Geometry: final body of the model. Coordinates: model frame, mm. Give positions to 0.01 mm unless a question says otherwise; leave off trailing zeros. Write each loop counter-clockwise with the first axis right and the second up, starting at its lowest first coordinate (ties: lowest second). Pieces come first, ordered by that corner, then holes. Notation, with made-up numbers: (-39.5, 20) -> (19.5, 20) arc R28 cw to (19.5, 54) -> close; hole circle Ø4 at (16, 24). An arc over 180 degrees is marked (long way). Answer as a JSON object with one key per item and string values.
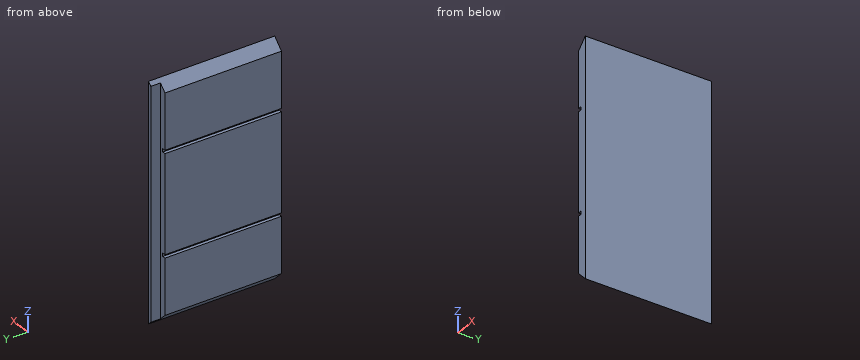
from build123d import *

# Parameters (mm, degrees)
F0_W     = 247.65
F0_H     = 457.2
F1_DEPTH = 19.05
F2_W     = 12.7
F2_H     = 19.05
F3_DEPTH = 457.201
F4_SIZE  = 19.04999
F5_SIZE  = 19.04999
F6_W     = 228.6
F6_H     = 6.35
F7_DEPTH = 6.35


# Not quite as in the source:
# - a fillet or chamfer is up to 0.001 mm smaller than in the source, because OpenCascade refuses the exact size


with BuildPart() as f1:
    # F0 (on Right) → F1 (new body)
    with BuildSketch(Plane.YZ):
        Rectangle(F0_W, F0_H)
    extrude(amount=F1_DEPTH)

    # F2 (on face) → F3 (cut, through all)
    with BuildSketch(Plane(origin=(0, 0, -228.6), x_dir=(1, 0, 0), z_dir=(0, 0, -1))):
        with Locations((6.35, -114.3)):
            Rectangle(F2_W, F2_H)
    extrude(amount=-F3_DEPTH, mode=Mode.SUBTRACT)

    # F4 (size 19.05 in the source; OpenCascade refuses exactly that, so slightly less here)
    f4_edges = [f1.edges().sort_by_distance(p)[0] for p in [
        (0, -9.525, 228.6),
    ]]
    chamfer(f4_edges, length=F4_SIZE)

    # F5 (size 19.05 in the source; OpenCascade refuses exactly that, so slightly less here)
    f5_edges = [f1.edges().sort_by_distance(p)[0] for p in [
        (0, -9.525, -228.6),
    ]]
    chamfer(f5_edges, length=F5_SIZE)

    # F6 (on face) → F7 (cut)
    with BuildSketch(Plane(origin=(0, 0, 0), x_dir=(0, -1, 0), z_dir=(-1, 0, 0))):
        with Locations((9.525, -98.425)):
            Rectangle(F6_W, F6_H)
        with Locations((9.525, 98.425)):
            Rectangle(F6_W, F6_H)
    extrude(amount=-F7_DEPTH, mode=Mode.SUBTRACT)


solid = f1.part
Q1. Cut plane B-B (z = -127). Return the cut outline in (x, y) (3 decimals).
Values:
{"outline": "(0, -123.825) -> (19.05, -123.825) -> (19.05, 123.825) -> (12.7, 123.825) -> (12.7, 104.775) -> (0, 104.775) -> close"}
Q2. First-contact query: P1, Ø3, axis at x = 2, y = -17, coming from the +Z side; P2, Ø3, axis at x = 4, y = 46, coming from the +Z side; P3, Ø7, axis at x = 3.5, y = 12.5, coming from the -Z side. Flat tips, straight axial feed; report the tip coordinate or a pass-through.
Values:
{"P1": "z = 213.05", "P2": "z = 215.05", "P3": "z = -216.55"}
Q3. Material intervals for L1, parallel to Z at x = 4, y = 0.5; L2, parallel to Z at x = 1.5, y = -60; L3, parallel to Y at x = 5.5, z = -129 (3 decimals), sorted ascending. Write a range as from..to.
Values:
{"L1": "-213.55..-101.6, -95.25..95.25, 101.6..213.55", "L2": "-211.05..-101.6, -95.25..95.25, 101.6..211.05", "L3": "-123.825..104.775"}
